Build history of the part. All positions in model axes, mm. A direction names the side the tool comes from. Give positions to 0.01 mm unless a question says otherwise; leave off trailing zeros. Loops run counter-clockwise (first coordinate to the right, second up) from the corner with the lowest first, then second, coordinate; pieces in that order, holes last.
1) Flat gauge pins, fed straight in: P1, Ø2.5, axis at x = 37.5, z = 23.5, coming from the +Y side; P2, Ø2, axis at x = 26, y = -50.5, coming from the -Z side; P3, Ø1.5, axis at x = 41, z = 37.5, coming from the -Y side. Where does each tip first touch, or does it go through?
2) Wall check: line 1 (Y direction, x = 30.5, z = 8.5); line 2 (X direction, y = -51, z = 8); line 3 (X direction, y = -23, z = 27.5). Give the ranges that are in metal, low to high.
3) Two-plate mould, pull along Y, no slides. Class faces 5 (the flat face through (51, -27, 6)), 6 (the flat face through (25, -8, 8)), 7 (the flat face through (26, -4, 34)): +Y half, -Y half, draft (parallel to the pull), parting line (faces both ways), or undercut.
4) Band-saw the part on C-C on z = 23. List the corners of the cut face in (x, y).
5) 3-axis set-ups, long thin cutter, end or side, ignore diameter. For faces 1 (the flat face through (25, -47, 8)), 2 (the flat face through (25, -53, 5)), 3 (the flat face through (8, -27, 0)), 4 (the flat face through (25, -6, 7)): which of +Z, -Z, +X, -X, +Y, -Y reach the whole face in a straight line?
6) Band-saw the part on B-B on y = -51. List the corners of the cut face in (x, z), then the cut area to 3 significant figures.
7) Band-saw the part on D-D on y = -42.5. List the corners of the cut face in (x, z), then the cut area to 3 significant figures.
8) Band-saw the part on A-A on x = 25.5. List the corners of the cut face in (y, z).
```python
from build123d import *

# Parameters (mm, degrees)
F0_W      = 20
F0_H      = 8
F1_DEPTH  = 12
F2_DEPTH  = 5
F3_DEPTH  = 5
F5_DEPTH  = 2
F4_R      = 2.25
F6_DEPTH  = 25
F8_DEPTH  = 2
F7_R      = 2.25
F9_DEPTH  = 25
F11_DEPTH = 30
F12_W     = 6
F12_H     = 30
F13_DEPTH = 4
F14_W     = 6
F14_H     = 30
F15_DEPTH = 4
F16_W     = 32
F16_H     = 47
F17_DEPTH = 9
F18_R     = 5
F18_R_2   = 2.5
F19_DEPTH = 7
F20_DEPTH = 25
F21_R     = 2.05
F22_DEPTH = 58
F23_DEPTH = 13
F24_DEPTH = 2


with BuildPart() as f1:
    # F0 (on Top) → F1 (new body)
    with BuildSketch(Plane.XY):
        with Locations((25.5, -4)):
            Rectangle(F0_W, F0_H)
        with Locations((25.5, -51)):
            Rectangle(F0_W, F0_H)
        with BuildLine():
            Line((6, 0), (0, 0))
            Line((0, 0), (0, -55))
            Line((0, -55), (6, -55))
            Line((6, -55), (6, -45.71))
            ThreePointArc((6, -45.71), (3.75, -43.46), (6, -41.21))
            Line((6, -41.21), (6, -32.98))
            ThreePointArc((6, -32.98), (3.75, -30.73), (6, -28.48))
            Line((6, -28.48), (6, -20.25))
            ThreePointArc((6, -20.25), (3.75, -18), (6, -15.75))
            Line((6, -15.75), (6, -7.52))
            ThreePointArc((6, -7.52), (3.75, -5.27), (6, -3.02))
            Line((6, -3.02), (6, 0))
        make_face()
        with BuildLine():
            Line((51, 0), (45, 0))
            Line((45, 0), (45, -3.02))
            ThreePointArc((45, -3.02), (46.5909902577, -3.6790097423), (47.25, -5.27))
            ThreePointArc((47.25, -5.27), (46.5909902577, -6.8609902577), (45, -7.52))
            Line((45, -7.52), (45, -15.75))
            ThreePointArc((45, -15.75), (46.5909902577, -16.4090097423), (47.25, -18))
            ThreePointArc((47.25, -18), (46.5909902577, -19.5909902577), (45, -20.25))
            Line((45, -20.25), (45, -28.48))
            ThreePointArc((45, -28.48), (46.5909902577, -29.1390097423), (47.25, -30.73))
            ThreePointArc((47.25, -30.73), (46.5909902577, -32.3209902577), (45, -32.98))
            Line((45, -32.98), (45, -41.21))
            ThreePointArc((45, -41.21), (46.5909902577, -41.8690097423), (47.25, -43.46))
            ThreePointArc((47.25, -43.46), (46.5909902577, -45.0509902577), (45, -45.71))
            Line((45, -45.71), (45, -55))
            Line((45, -55), (51, -55))
            Line((51, -55), (51, 0))
        make_face()
        with BuildLine():
            Line((15.5, 0), (6, 0))
            Line((6, 0), (6, -3.02))
            ThreePointArc((6, -3.02), (7.5909902577, -3.6790097423), (8.25, -5.27))
            ThreePointArc((8.25, -5.27), (7.5909902577, -6.8609902577), (6, -7.52))
            Line((6, -7.52), (6, -15.75))
            ThreePointArc((6, -15.75), (7.5909902577, -16.4090097423), (8.25, -18))
            ThreePointArc((8.25, -18), (7.5909902577, -19.5909902577), (6, -20.25))
            Line((6, -20.25), (6, -28.48))
            ThreePointArc((6, -28.48), (7.5909902577, -29.1390097423), (8.25, -30.73))
            ThreePointArc((8.25, -30.73), (7.5909902577, -32.3209902577), (6, -32.98))
            Line((6, -32.98), (6, -41.21))
            ThreePointArc((6, -41.21), (7.5909902577, -41.8690097423), (8.25, -43.46))
            ThreePointArc((8.25, -43.46), (7.5909902577, -45.0509902577), (6, -45.71))
            Line((6, -45.71), (6, -55))
            Line((6, -55), (15.5, -55))
            Line((15.5, -55), (15.5, -47))
            Line((15.5, -47), (15.5, -35))
            Line((15.5, -35), (12.5, -35))
            Line((12.5, -35), (12.5, -9.5))
            Line((12.5, -9.5), (15.5, -9.5))
            Line((15.5, -9.5), (15.5, -8))
            Line((15.5, -8), (15.5, 0))
        make_face()
        with BuildLine():
            Line((45, 0), (35.5, 0))
            Line((35.5, 0), (35.5, -8))
            Line((35.5, -8), (35.5, -9.5))
            Line((35.5, -9.5), (38.5, -9.5))
            Line((38.5, -9.5), (38.5, -35))
            Line((38.5, -35), (35.5, -35))
            Line((35.5, -35), (35.5, -47))
            Line((35.5, -47), (35.5, -55))
            Line((35.5, -55), (45, -55))
            Line((45, -55), (45, -45.71))
            ThreePointArc((45, -45.71), (42.75, -43.46), (45, -41.21))
            Line((45, -41.21), (45, -32.98))
            ThreePointArc((45, -32.98), (42.75, -30.73), (45, -28.48))
            Line((45, -28.48), (45, -20.25))
            ThreePointArc((45, -20.25), (42.75, -18), (45, -15.75))
            Line((45, -15.75), (45, -7.52))
            ThreePointArc((45, -7.52), (42.75, -5.27), (45, -3.02))
            Line((45, -3.02), (45, 0))
        make_face()
    extrude(amount=F1_DEPTH)

    # F0 (on Top) → F2 (cut)
    with BuildSketch(Plane.XY):
        with Locations((25.5, -51)):
            Rectangle(F0_W, F0_H)
    extrude(amount=F2_DEPTH, mode=Mode.SUBTRACT)

    # F0 (on Top) → F3 (cut)
    with BuildSketch(Plane.XY):
        with Locations((25.5, -4)):
            Rectangle(F0_W, F0_H)
    extrude(amount=F3_DEPTH, mode=Mode.SUBTRACT)

    # F4 (on face) → F5 (cut)
    with BuildSketch(Plane(origin=(0, 0, 5), x_dir=(1, 0, 0), z_dir=(0, 0, -1))):
        Polygon((24.5, 47), (25.5, 47), (26.5, 47), (26.5, 52), (24.5, 52), align=None)
    extrude(amount=-F5_DEPTH, mode=Mode.SUBTRACT)

    # F4 (on face) → F6 (cut)
    with BuildSketch(Plane(origin=(0, 0, 5), x_dir=(1, 0, 0), z_dir=(0, 0, -1))):
        with Locations((20.5, 51)):
            Circle(F4_R)
        with Locations((30.5, 51)):
            Circle(F4_R)
    extrude(amount=-F6_DEPTH, mode=Mode.SUBTRACT)

    # F7 (on face) → F8 (cut)
    with BuildSketch(Plane(origin=(0, 0, 5), x_dir=(1, 0, 0), z_dir=(0, 0, -1))):
        Polygon((26.5, 8), (25.5, 8), (24.5, 8), (24.5, 3), (26.5, 3), align=None)
    extrude(amount=-F8_DEPTH, mode=Mode.SUBTRACT)

    # F7 (on face) → F9 (cut)
    with BuildSketch(Plane(origin=(0, 0, 5), x_dir=(1, 0, 0), z_dir=(0, 0, -1))):
        with Locations((30.5, 4)):
            Circle(F7_R)
        with Locations((20.5, 4)):
            Circle(F7_R)
    extrude(amount=-F9_DEPTH, mode=Mode.SUBTRACT)

    # F10 (on face) → F11 (join)
    with BuildSketch(Plane.XY.offset(12)):
        Polygon((41.5, -55), (41.5, 0), (35.5, 0), (35.5, -8), (35.5, -9.5), (38.5, -9.5), (38.5, -35), (35.5, -35), (35.5, -47), (35.5, -55), align=None)
        Polygon((15.5, -8), (15.5, 0), (9.5, 0), (9.5, -55), (15.5, -55), (15.5, -47), (15.5, -35), (12.5, -35), (12.5, -9.5), (15.5, -9.5), align=None)
    extrude(amount=F11_DEPTH)

    # F12 (on face) → F13 (cut)
    with BuildSketch(Plane(origin=(0, 0, 0), x_dir=(-1, 0, 0), z_dir=(0, 1, 0))):
        with Locations((-38.5, 27)):
            Rectangle(F12_W, F12_H)
        with Locations((-12.5, 27)):
            Rectangle(F12_W, F12_H)
    extrude(amount=-F13_DEPTH, mode=Mode.SUBTRACT)

    # F14 (on face) → F15 (cut)
    with BuildSketch(Plane.XZ.offset(55)):
        with Locations((12.5, 27)):
            Rectangle(F14_W, F14_H)
        with Locations((38.5, 27)):
            Rectangle(F14_W, F14_H)
    extrude(amount=-F15_DEPTH, mode=Mode.SUBTRACT)

    # F16 (on face) → F17 (join)
    with BuildSketch(Plane.XY.offset(42)):
        with Locations((25.5, -27.5)):
            Rectangle(F16_W, F16_H)
    extrude(amount=-F17_DEPTH)

    # F18 (on face) → F19 (cut)
    with BuildSketch(Plane.XY.offset(42)):
        with Locations((25.5, -18)):
            Circle(F18_R)
        with Locations((25.5, -18)):
            Circle(F18_R_2, mode=Mode.SUBTRACT)
    extrude(amount=-F19_DEPTH, mode=Mode.SUBTRACT)

    # F20 (cut): a face of the model
    f20_faces = [f1.faces().sort_by_distance(p)[0] for p in [
        (25.5, -18, 42),
    ]]
    extrude(f20_faces, amount=-F20_DEPTH, mode=Mode.SUBTRACT)

    # F21 (on face) → F22 (cut)
    with BuildSketch(Plane.YZ.offset(41.5)):
        with Locations((-18, 38.5)):
            Circle(F21_R)
    extrude(amount=-F22_DEPTH, mode=Mode.SUBTRACT)

    # F23 (cut): a face of the model
    f23_faces = [f1.faces().sort_by_distance(p)[0] for p in [
        (41.061365756, -51, 27),
    ]]
    extrude(f23_faces, amount=-F23_DEPTH, mode=Mode.SUBTRACT)

    # F24 (add): a face of the model
    f24_faces = [f1.faces().sort_by_distance(p)[0] for p in [
        (25.5, 0, 6.68359375),
    ]]
    extrude(f24_faces, amount=F24_DEPTH)


solid = f1.part
```
Findings below:
1. P1: stops at y = -4
1. P2: stops at z = 5
1. P3: stops at y = -38
2. line 1: y = -55 to -53.25, -48.75 to -47, -8 to -6.25, -1.75 to 2
2. line 2: x = 0 to 18.25, 22.75 to 28.25, 32.75 to 51
2. line 3: x = 9.5 to 12.5, 38.5 to 41.5
3. face 5: draft
3. face 6: undercut
3. face 7: +Y half
4. outline: (9.5, -38) - (15.5, -38) - (15.5, -35) - (12.5, -35) - (12.5, -9.5) - (15.5, -9.5) - (15.5, -4) - (9.5, -4) - close; (35.5, -38) - (41.5, -38) - (41.5, -4) - (35.5, -4) - (35.5, -9.5) - (38.5, -9.5) - (38.5, -35) - (35.5, -35) - close
5. face 1: +Z, -Z
5. face 2: -Z, +Y, -Y
5. face 3: -Z, +X, -X, +Y, -Y
5. face 4: -Z
6. outline: (0, 0) - (15.5, 0) - (15.5, 5) - (18.25, 5) - (18.25, 12) - (0, 12) - close; (22.75, 5) - (24.5, 5) - (24.5, 7) - (26.5, 7) - (26.5, 5) - (28.25, 5) - (28.25, 12) - (22.75, 12) - close; (32.75, 5) - (35.5, 5) - (35.5, 0) - (51, 0) - (51, 12) - (32.75, 12) - close
6. area: 445 mm2
7. outline: (0, 0) - (3.97, 0) - (3.97, 12) - (0, 12) - close; (8.03, 0) - (15.5, 0) - (15.5, 12) - (8.03, 12) - close; (35.5, 0) - (42.97, 0) - (42.97, 12) - (35.5, 12) - close; (47.03, 0) - (51, 0) - (51, 12) - (47.03, 12) - close
7. area: 274 mm2
8. outline: (-55, 5) - (-52, 5) - (-52, 7) - (-47, 7) - (-47, 12) - (-55, 12) - close; (-38, 33) - (-20.5, 33) - (-20.5, 35) - (-23, 35) - (-23, 42) - (-38, 42) - close; (-15.5, 33) - (-4, 33) - (-4, 42) - (-13, 42) - (-13, 35) - (-15.5, 35) - close; (-8, 7) - (-3, 7) - (-3, 5) - (2, 5) - (2, 12) - (-8, 12) - close
